Geometry: see drawing. Coordinates: mm, zero at the bounding-box minimum. Round coordinates to 2 decimals unless told otherwise and drop trailing zeros. Loops run counter-clockwise (first coordinate to the right, second up) from the corner with the lowest first, then second, coordinate; pieces in that order, holes last. Notation, with made-up numbers: M 89,84.25 L 127,84.25 A12 cw 127,94.25 Z; hole C -5,72.5 d11. An arc over 180 degrees is marked long. Answer as a JSON object with one key per item and string values.
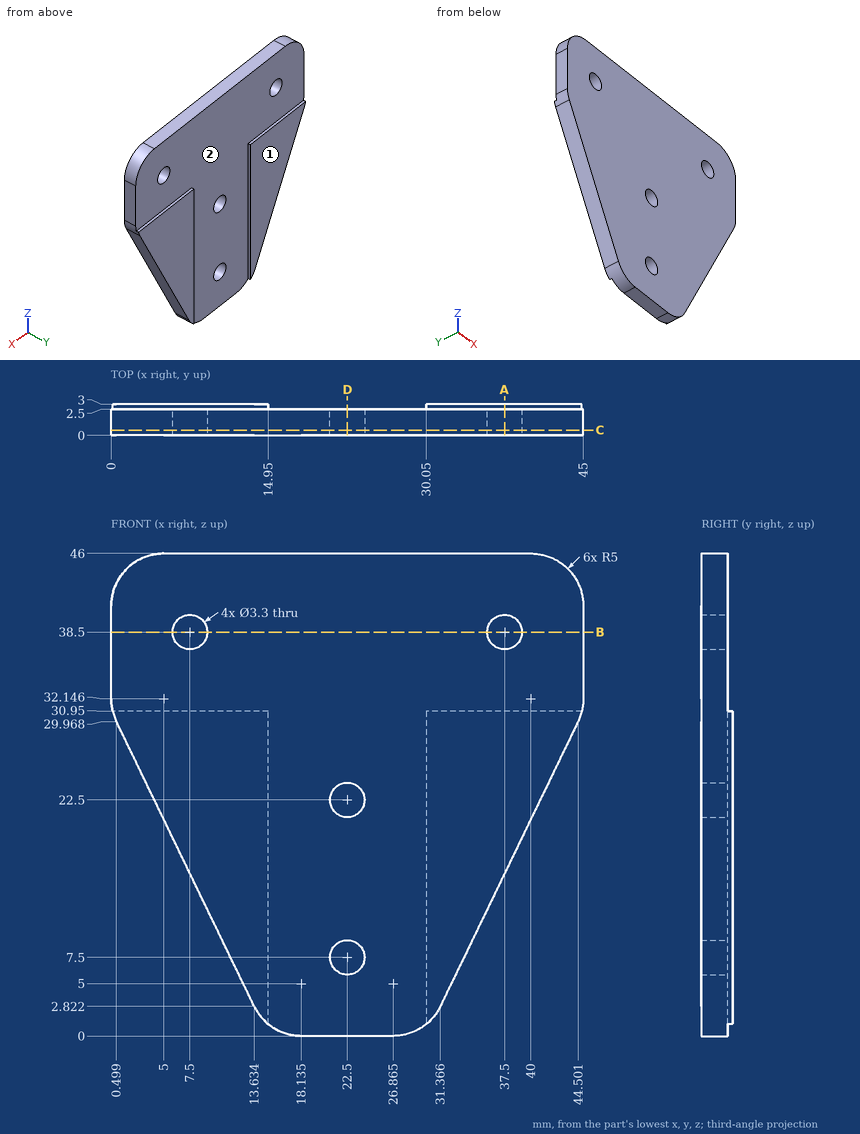
1) Section query B-B (z = 38.5). Return the cut outline in (x, y).
Results:
{"outline": "M 0,0 L 5.85,0 L 5.85,2.5 L 0,2.5 Z; M 9.15,0 L 35.85,0 L 35.85,2.5 L 9.15,2.5 Z; M 39.15,0 L 45,0 L 45,2.5 L 39.15,2.5 Z"}
2) Section query A-A (x = 37.5). Return the cut outline in (y, z).
Results:
{"outline": "M 0,15.5 L 3,15.5 L 3,30.95 L 2.5,30.95 L 2.5,36.85 L 0,36.85 Z; M 0,40.15 L 2.5,40.15 L 2.5,46 L 0,46 Z"}
3) Section query D-D (x = 22.5). Return the cut outline in (y, z).
Results:
{"outline": "M 0,0 L 2.5,0 L 2.5,5.85 L 0,5.85 Z; M 0,9.15 L 2.5,9.15 L 2.5,20.85 L 0,20.85 Z; M 0,24.15 L 2.5,24.15 L 2.5,46 L 0,46 Z"}
4) Section query C-C (y = 0.5). Count the separate pieces of the cut face and the enclosed holes in it, and give its area (3 significant figures).
Results:
{"separate pieces": "1", "enclosed holes": "4", "area": "1,560 mm2"}
5) Pin query (flat end, axial travel): P1, Ø4, axis at x = 7.5, z = 38.5, coming from the +Y side; P2, Ø1.5, axis at y = 1.5, z = 28, coming from the +X side; P3, Ø2, axis at x = 22.5, z = 7.5, coming from the -Y side. Return the tip coordinate at first contact, or that it passes through.
Results:
{"P1": "y = 2.5", "P2": "x = 43.91", "P3": "through"}
6) Pull-direction query (X, two-part tool) for the marked faces 1 and 2; classes: +X half, -X half, draft (parallel to the pull), parting line (faces both ways), or undercut.
Results:
{"face 1": "draft", "face 2": "undercut"}
7) Ray query, line 1 (X direction, y = 1.05, z = 38.5); line 2 (Z direction, x = 22.5, y = 1); line 3 (Y direction, x = 23, z = 11). Return the intervals inside material, ascending.
Results:
{"line 1": "0 to 5.85, 9.15 to 35.85, 39.15 to 45", "line 2": "0 to 5.85, 9.15 to 20.85, 24.15 to 46", "line 3": "0 to 2.5"}
